Input: dimensioned drawing with shaded views. Units: mm. Origin: part minimum x, y, z. A direction names the side the tool comes from. Give positions to 0.01 mm unless a question says otherwise; leave off trailing zeros. Order: outer loops, then holes, each group sorted by start corner. A loop starts at its lowest first (then second) coordinate and runs counter-clockwise, first axis right, second up. Notation, with made-up numbers: (22, -20) -> (56, -20) arc R26 cw to (56, 12) -> close; hole circle Ø7 at (61.5, 36.25). An arc over 180 degrees is marked (long way). Use CSV: the item, a comma, the result in double quotes.
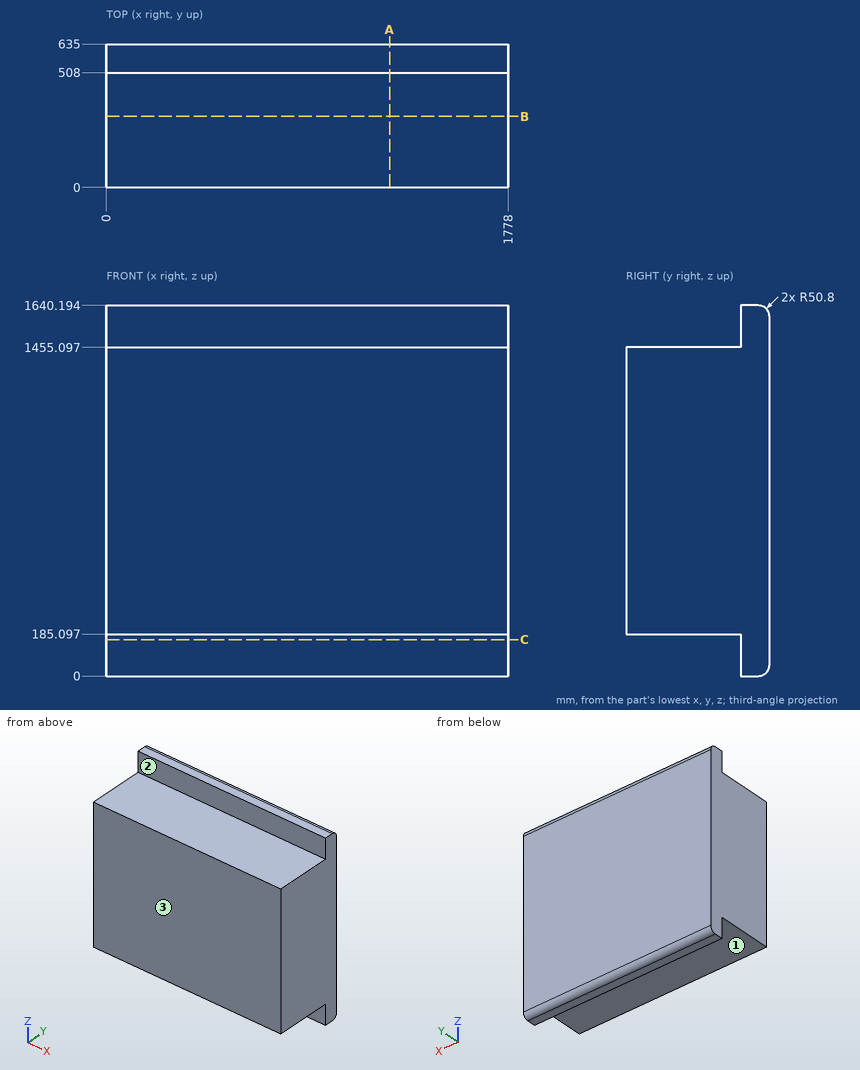
1. Pin query (flat end, axial travel): P1, Ø2, axis at x = 1192.5, y = 505.5, coming from the +Z side. Return the tip coordinate at first contact, or that it passes through.
Answer below:
P1,"stops at z = 1455.1"
2. Access query for the marked faces 1, 2 and 3. Directions: +Z, -Z, +X, -X, +Y, -Y. A direction counts if a zero-diameter tool reaches every point of the face in a straight line with its end or side. Return the directions, or none.
Answer below:
face 1,"-Z, +X, -X, -Y"
face 2,"+Z, +X, -X, -Y"
face 3,"+Z, -Z, +X, -X, -Y"
3. Section query A-A on x = 1253.5. Return loops of the section in (y, z), plus the area to 3 significant figures.
Answer below:
outline,"(0, 185.1) -> (508, 185.1) -> (508, 0) -> (584.2, 0) arc R50.8 ccw to (635, 50.8) -> (635, 1589.39) arc R50.8 ccw to (584.2, 1640.19) -> (508, 1640.19) -> (508, 1455.1) -> (0, 1455.1) -> close"
area,"852,000 mm²"
4. Ray query, line 1 along Z through (x, y) = (360, 57.5); line 2 along Y through (x, z) = (1150.5, 134). Return the intervals inside material, ascending.
Answer below:
line 1,"z = 185.1 to 1455.1"
line 2,"y = 508 to 635"
5. Section query B-B on y = 315. Return loops of the section in (x, z).
Answer below:
outline,"(0, 185.1) -> (1778, 185.1) -> (1778, 1455.1) -> (0, 1455.1) -> close"
6. Section query C-C on z = 160.5. Return loops of the section in (x, y).
Answer below:
outline,"(0, 508) -> (1778, 508) -> (1778, 635) -> (0, 635) -> close"
